Build history of the part. All positions in model axes, mm. A direction names the side the tool comes from. Round coordinates to 2 decimals unless told otherwise and drop trailing zeros. Write each loop counter-clockwise with the first axis right and the second up, starting at its lowest first coordinate (ties: lowest second). Pieces come first, ordered by that corner, then holes. Notation, with made-up numbers: (37, 77) -> (90, 77) arc R24 ccw to (90, 92) -> close; hole circle Ø2 at (73.25, 20.5). An arc over 180 degrees is marked (long way). Answer in a Markdown table with one row per item. Add a question column.
from build123d import *

# Parameters (mm, degrees)
CROQUIS1_R              = 10
CROQUIS1_R_2            = 1.5
CROQUIS1_R_3            = 1.533499393
CROQUIS1_R_4            = 2.75
SALIENTE_EXTRUIR1_DEPTH = 2
CROQUIS2_R              = 4.75
CROQUIS2_R_2            = 2.85
SALIENTE_EXTRUIR2_DEPTH = 3.5


with BuildPart() as part:
    # Croquis1 → Saliente-Extruir1 (new body)
    # profile 1 of 2: a face of its own
    with BuildSketch(Plane(origin=(0, 0, 0), x_dir=(1, 0, 0), z_dir=(0, 1, 0))):
        with Locations(Location((0, 0, 0), (0, 0, 270))):
            Circle(CROQUIS1_R)
        with Locations(Location((-7, 0, 0), (0, 0, 270))):
            Circle(CROQUIS1_R_2, mode=Mode.SUBTRACT)
        with Locations(Location((0, -7, 0), (0, 0, 270))):
            Circle(CROQUIS1_R_2, mode=Mode.SUBTRACT)
        with Locations(Location((7, 0, 0), (0, 0, 270))):
            Circle(CROQUIS1_R_2, mode=Mode.SUBTRACT)
        with Locations(Location((0, 7, 0), (0, 0, 270))):
            Circle(CROQUIS1_R_3, mode=Mode.SUBTRACT)
        Circle(CROQUIS1_R_4, mode=Mode.SUBTRACT)
    # profile 2 of 2: a face of its own
    with BuildSketch(Plane(origin=(0, 0, 0), x_dir=(1, 0, 0), z_dir=(0, 1, 0))):
        Circle(CROQUIS1_R_4)
        with Locations(Location((0, 0, 0), (0, 0, 270))):
            Circle(CROQUIS1_R_2, mode=Mode.SUBTRACT)
    extrude(amount=SALIENTE_EXTRUIR1_DEPTH)

    # Croquis2 → Saliente-Extruir2 (add)
    with BuildSketch(Plane(origin=(0, 2, 0), x_dir=(1, 0, 0), z_dir=(0, 1, 0))):
        with Locations(Location((0, 0, 0), (0, 0, 270))):
            Circle(CROQUIS2_R)
        with Locations(Location((0, 0, 0), (0, 0, 270))):
            Circle(CROQUIS2_R_2, mode=Mode.SUBTRACT)
    extrude(amount=SALIENTE_EXTRUIR2_DEPTH)


solid = part.part
(1) Saw through at D-D (x = 7). List the corners of the cut face in (y, z).
(2) Drop flat-ended pins along their axis: P1, Ø2.5, axis at x = 7, z = 0, coming from the +Y side; P2, Ø2, axis at x = -3, y = 2.5, coming from the +Z side; P3, Ø4, axis at x = 0, z = 0, coming from the +Y side. Give the stop position or say it passes through.
(3) Which spindle directions (+Z, -Z, +X, -X, +Y, -Y) get a long thin tool onto all of the face, cutting with end or side? Do faces 4 (the face through (0.45, 0.99, 1.43)), 5 (the face through (-1.734, 3.726, -2.262)). Say none if no direction does.
(4) Saw through at B-B (x = 0). List the corners of the cut face in (y, z).
(5) Mould opens along X. For faces 1 (the face through (0.07, 0.99, 5.5)), 2 (the face through (-2.89, 3.73, -3.77)), 3 (the face through (4.3, 2, -2.4)) say: pulls with the +X half, pulls with the -X half, needs draft (parallel to the pull), parting line crosses it, or undercut.
(6) Saw through at A-A (y = 1.25). List the corners of the cut face in (x, z).
(7) Saw through at C-C (z = -7.75). List the corners of the cut face in (x, y), plus the area to 3 significant figures.
(8) Probe line 1 along X through (y, z) = (1.1, 0); line 2 along X through (y, z) = (3.8, 0); line 3 along Y through (x, z) = (2.25, -5.5). List the from-to ranges inside material, lowest first.
Answer sheet:
| question | item | result |
|---|---|---|
| 1 | outline | (0, -7.14) -> (2, -7.14) -> (2, -1.5) -> (0, -1.5) -> close; (0, 1.5) -> (2, 1.5) -> (2, 7.14) -> (0, 7.14) -> close |
| 2 | P1 | passes through |
| 2 | P2 | stops at z = 9.77 |
| 2 | P3 | stops at y = 2 |
| 3 | face 4 | +Y, -Y |
| 3 | face 5 | +Y |
| 4 | outline | (0, -10) -> (2, -10) -> (2, -8.53) -> (0, -8.53) -> close; (0, -5.47) -> (2, -5.47) -> (2, -4.75) -> (5.5, -4.75) -> (5.5, -2.85) -> (2, -2.85) -> (2, -1.5) -> (0, -1.5) -> close; (0, 1.5) -> (2, 1.5) -> (2, 2.85) -> (5.5, 2.85) -> (5.5, 4.75) -> (2, 4.75) -> (2, 5.5) -> (0, 5.5) -> close; (0, 8.5) -> (2, 8.5) -> (2, 10) -> (0, 10) -> close |
| 5 | face 1 | undercut |
| 5 | face 2 | parting line crosses it |
| 5 | face 3 | needs draft |
| 6 | outline | circle Ø20 at (0, 0); hole circle Ø3 at (-7, 0); hole circle Ø3.07 at (0, -7); hole circle Ø3 at (0, 0); hole circle Ø3 at (0, 7); hole circle Ø3 at (7, 0) |
| 7 | outline | (-6.32, 0) -> (-1.34, 0) -> (-1.34, 2) -> (-6.32, 2) -> close; (1.34, 0) -> (6.32, 0) -> (6.32, 2) -> (1.34, 2) -> close |
| 7 | area | 19.9 mm² |
| 8 | line 1 | x = -10 to -8.5, -5.5 to -1.5, 1.5 to 5.5, 8.5 to 10 |
| 8 | line 2 | x = -4.75 to -2.85, 2.85 to 4.75 |
| 8 | line 3 | y = 0 to 2 |
